Autodesk Inventor part; units mm, degrees
ref_plane "bolt_XY" through (0, 0, 0) normal (1, 0, 0) x (0, 0, -1)
ref_plane "bolt_YZ" through (0, 0, 0) normal (0, 0, -1) x (0, 1, 0)
ref_plane "bolt_ZX" through (0, 0, 0) normal (0, 1, 0) x (1, 0, 0)
sketch "Sketch_2" plane through (0, 0, 0) normal (0, 0, 1) x (1, 0, 0)
  line L0 (30, 0) -> (-5, 0)
  line L1 (-5, 0) -> (-5, 3.6833)
  line L2 (-5, 3.6833) -> (-4.4333, 4.25)
  line L3 (-4.4333, 4.25) -> (0, 4.25)
  line L4 (0, 4.25) -> (0, 2.5)
  line L5 (0, 2.5) -> (29.5085, 2.5)
  line L6 (29.5085, 2.5) -> (30, 2.0085)
  line L7 (30, 2.0085) -> (30, 0)
  line L8 (30, 0) -> (-5, 0)
revolve "Revolution1" add sketch "Sketch_2" angle 360 about axis through (30, 0, 0) along (1, 0, 0)
thread "Thread1"
sketch "Sketch_4" plane through (0, 0, 0) normal (0, 0, 1) x (1, 0, 0)
  line L0 (-1.9641, 0) -> (-5, 0)
  line L1 (-5, 0) -> (-5, 2)
  line L2 (-5, 2) -> (-2.5, 2)
  line L3 (-2.5, 2) -> (-1.9641, 0)
  line L4 (-1.9641, 0) -> (-5, 0)
revolve "Revolution2" cut sketch "Sketch_4" angle 360 about axis through (-1.9641, 0, 0) along (1, 0, 0)
sketch "Sketch_3" plane through (-5, 0, 0) normal (1, 0, 0) x (0, 0, -1)
  line L0 (-2, 1.1547) -> (-2, -1.1547)
  line L1 (-2, -1.1547) -> (0, -2.3094)
  line L2 (0, -2.3094) -> (2, -1.1547)
  line L3 (2, -1.1547) -> (2, 1.1547)
  line L4 (2, 1.1547) -> (0, 2.3094)
  line L5 (0, 2.3094) -> (-2, 1.1547)
extrude "Extrusion1" cut sketch "Sketch_3" along normal blind 2.5
ref_plane "bolt_XY" through (0, 0, 0) normal (1, 0, 0) x (0, 0, -1)
ref_plane "bolt_YZ" through (0, 0, 0) normal (0, 0, -1) x (0, 1, 0)
ref_plane "bolt_ZX" through (0, 0, 0) normal (0, 1, 0) x (1, 0, 0)
ref_plane "nut_XY" through (30, 0, 0) normal (1, 0, 0) x (0, 0, -1)
ref_plane "nut_YZ" through (30, 0, 0) normal (0, 0, -1) x (0, 1, 0)
ref_plane "nut_ZX" through (30, 0, 0) normal (0, 1, 0) x (1, 0, 0)
properties part number "CBM5-30" material "MISUMI"
The listing builds one solid part. Answer for the finished solid, in the listing's coordinates (mm). A direction names the side the tool comes from. Give positions to 0.01 mm unless a question says otherwise; leave off trailing zeros. Loops run counter-clockwise (first coordinate to the right, second up) from the corner with the lowest first, then second, coordinate; pieces in that order, holes last.
Item 1: Determine the mould class of faces 4 (the flat face through (-5, 2, -2)), 5 (the flat face through (-3.768, -1.724, 1.014)), 6 (the cylindrical face through (-2.186, 2.285, 3.584)) for opening direction Y: +Y half, -Y half, draft (parallel to the pull), parting line (faces both ways), or undercut.
Derived:
face 4: draft
face 5: undercut
face 6: parting line
Item 2: Each of these flat-tipped pins is pushed along its axis until it touches: pin 1 Ø1.1 at (y, z) = (-0.5, 1.5) entering from -X; pin 2 Ø5 at (x, y) = (22, 0) entering from -Z; pin 3 Ø2 at (x, z) = (23.5, 0.5) entering from -Y; pin 4 Ø1.5 at (x, y) = (4.5, 0.5) entering from +Z. Where does it stop, or does it pass through?
Derived:
pin 1: stops at x = -5
pin 2: stops at z = -2.5
pin 3: stops at y = -2.5
pin 4: stops at z = 2.5
Item 3: Find the intervals of material crossed by line 1 along X through (y, z) = (-2, -1.75); line 2 along Z through (x, y) = (8.5, 1.5), in increasing order.
Derived:
line 1: x = -5 to 0
line 2: z = -2 to 2
Item 4: A tool of negligible diameter and unlimited length cuts with its end or side. For faces 1 (the flat face through (-3.77, 1.74, 0.99)), 2 (the flat face through (30, 0, 0)), 3 (the flat face through (0, 2, -2)), from which of +Z, -Z, +X, -X, +Y, -Y can it reach the whole face along a straight path? Write none if from no direction.
Derived:
face 1: -X
face 2: +Z, -Z, +X, +Y, -Y
face 3: +X
Item 5: A cutting plane is placed at A-A (x = 8.5). Give the vertices of the cut face in (y, z), then the cut area to 3 significant figures.
Derived:
outline: circle Ø5 at (0, 0)
area: 19.6 mm2
